The model under review builds one solid part; all positions refer to its coordinate system, in mm. A direction names the side the tool comes from. Round coordinates to 2 decimals unless told otherwise and drop trailing zeros. Loops run counter-clockwise (first coordinate to the right, second up) from the corner with the lowest first, then second, coordinate; pieces in that order, holes last. Notation, with made-up numbers: (45, 60) - (62, 60) arc R26 cw to (62, 79) - close; hole circle Ø1 at (71, 76). An arc over 180 degrees is marked (long way). Answer as CSV lines item,"result".
Autodesk Inventor part; units mm, degrees
ref_plane "Work Plane1" through (34.8277, 0, 0) normal (0, 0, -1) x (1, 0, 0)
ref_plane "YZ Plane" through (0, 0, 0) normal (1, 0, 0) x (0, 1, 0)
ref_plane "XZ Plane" through (0, 0, 0) normal (0, 1, 0) x (-1, 0, 0)
sketch "Sketch1" plane through (0, 0, 0) normal (0, 0, 1) x (1, 0, 0)
  line L0 (0, 0) -> (8.636, 0)
  line L1 (0, 0) -> (0, 5.969)
  line L2 (8.636, 5.207) -> (8.636, 0)
  line L3 (0, 5.969) -> (5.7845, 12.9962)
  line L4 (8.636, 5.207) -> (9.4615, 5.207)
  arc A0 (9.4615, 5.207) -> (5.7845, 12.9962) centre (9.4615, 9.9695) ccw
  line L5 (8.636, 5.207) -> (0, 5.969)
  line L6 (8.636, 5.207) -> (0, 5.207)
  dimension "d0" = 10.414
  dimension "d1" = 9.4615
  dimension "d2" = 9.9695
  dimension "d3" = 4.7625
  dimension "d4" = 8.636
  dimension "d5" = 11.938
revolve "Body" add sketch "Sketch1" angle 360 about axis through (0, 0, 0) along (1, 0, 0) contours L1 L6 L2 L0 | L1 L5 L6
extrude "Wing1" add sketch "Sketch1" along normal mid plane 4.318 contours L1 L5 L6 | L5 L3 A0 L4
fillet "Fillet1" [suppressed]
mirror "Wing2" about plane through (0, 0, 0) normal (0, 1, 0) of "Wing1"
sketch "Sketch2" plane through (0, 0, 0) normal (1, 0, 0) x (0, 1, 0)
  line L0 (0, -14) -> (0, 14)
  line L1 (-14, 0) -> (14, 0)
  point P0 (0, 0)
hole "Thread" at (0, 0, 0) direction (1, 0, 0) diameter 4.9784 end through all
chamfer "Chamfer1" distance 0.6874 angle 30 1 edges at (0, 0, -2.4892) measured on face at (0, -4.5336, 0.1)
ref_plane "Work Plane1" through (34.8277, 0, 0) normal (0, 0, -1) x (1, 0, 0)
equation "\"d0\" = KOD2"
equation "\"d1\" = KOH1 - RR"
equation "\"d2\" = 0.5 * E0 - RR"
equation "\"d3\" = RR"
equation "\"d4\" = KOH"
equation "\"d5\" = KOD"
equation "\"d6\" = SW"
equation "\"d8\" = 0.333333 * SW"
equation "\"d9\" = -0.5 * GD1 + 0.5 * NND"
equation "\"d109\" = -0.5 * GD1 + 0.5 * NND"
equation "\"NND\" = 6.35"
equation "\"KOH\" = 8.636"
equation "\"KOH1\" = 14.224"
equation "\"SW\" = 4.318"
equation "\"KOD\" = 11.938"
equation "\"KOD2\" = 10.414"
equation "\"RR\" = 4.7625"
equation "\"E0\" = 29.464"
equation "\"THREADDIA\" = 6.35"
equation "\"TOA\" = 30deg"
equation "\"RR2\" = 1.905"
equation "\"SW1\" = SW"
properties part number "ANSI B18.17 - 1/4 - 20, TBS1WNI" material "Steel, Mild"
1. Take a section at C-C (x = 4.5). State the section outline as (y, z) points, plus the area to 3 significant figures.
Numbers:
outline,"(-11.44, -2.16) - (-5.21, -2.16) - (-5.21, -1.98) arc R5.57 ccw to (5.21, -1.98) - (5.21, -2.16) - (11.44, -2.16) - (11.44, 2.16) - (5.21, 2.16) - (5.21, 1.98) arc R5.57 ccw to (-5.21, 1.98) - (-5.21, 2.16) - (-11.44, 2.16) - close; hole circle Ø4.98 at (0, 0)"
area,"130 mm²"
2. Take a section at B-B (x = 7.75). State the section outline as (y, z) points.
Numbers:
outline,"(-14.41, -2.16) - (-5.21, -2.16) - (-5.21, -0.91) arc R5.29 ccw to (5.21, -0.91) - (5.21, -2.16) - (14.41, -2.16) - (14.41, 2.16) - (5.21, 2.16) - (5.21, 0.91) arc R5.29 ccw to (-5.21, 0.91) - (-5.21, 2.16) - (-14.41, 2.16) - close; hole circle Ø4.98 at (0, 0)"
3. Wall thickness on probe 1 along Z at (x, y) = (3.25, 9.75); probe 2 along Z at (x, y) = (4, 0); probe 3 along Y at (x, z) = (6.5, 0): over which ranges is each line inside the solid? List them lowest first.
Numbers:
probe 1,"z = -2.16 to 2.16"
probe 2,"z = -5.62 to -2.49, 2.49 to 5.62"
probe 3,"y = -13.7 to -2.49, 2.49 to 13.7"
4. Draft analysis for pull direction Y (two halves, no side actions). For faces 3 (the face through (9, 5.207, -1)), 4 (the face through (2.85, 9.43, -0.03)), 5 (the face through (4.574, -0.748, 2.374)), 6 (the face through (9, -9, -2.159)), state which applies: +Y half, -Y half, draft (parallel to the pull), parting line (faces both ways), or undercut.
Numbers:
face 3,"undercut"
face 4,"+Y half"
face 5,"undercut"
face 6,"draft"
5. Take a section at A-A (y = 0). State the section outline as (x, z) points.
Numbers:
outline,"(0, -5.97) - (8.64, -5.21) - (8.64, -2.49) - (0.4, -2.49) - (0, -3.18) - close; (0, 3.18) - (0.4, 2.49) - (8.64, 2.49) - (8.64, 5.21) - (0, 5.97) - close"
6. Take a section at D-D (y = 7.25). State the section outline as (x, z) points.
Numbers:
outline,"(1.05, -2.16) - (13.37, -2.16) - (13.37, 2.16) - (1.05, 2.16) - close"
7. Tool access review of faces 1 (the face through (8.636, -2.4, -1.1)), 2 (the face through (2.93, -9.53, -0.03)): name each direction out of +Z, -Z, +X, -X, +Y, -Y from which nothing blocks a thin tool from reaching the whole face with its end or side.
Numbers:
face 1,"+Z, -Z, +X"
face 2,"+Z, -Z, -X, -Y"
8. Clearance check with flat-ended pins moving along their axes: pin 1 (3 mm diameter, centred on x = 9, y = 11.5, fed in from +Z); pin 2 (1.5 mm diameter, centred on x = 7.5, y = -8, fed in from -Z); pin 3 (3.5 mm diameter, centred on x = 6.5, z = 0.5, fed in from +Y). State where each tip first meets the part, or that it passes through.
Numbers:
pin 1,"stops at z = 2.16"
pin 2,"stops at z = -2.16"
pin 3,"stops at y = 14.58"
